from build123d import *

# Parameters (mm, degrees)
SKETCH1_W           = 25.4
SKETCH1_H           = 69.85
SKETCH1_R           = 3.175
BOSS_EXTRUDE1_DEPTH = 6.35
FILLET1_R           = 12.7
FILLET2_R           = 2.116666667
SKETCH5_R           = 9.525
SKETCH5_R_2         = 7.016807895
CUT_EXTRUDE2_DEPTH  = 3.571875
SKETCH5_2_R         = 7.016807895
CUT_EXTRUDE3_DEPTH  = 6.35


with BuildPart() as part:
    # Sketch1 → Boss-Extrude1 (new body)
    with BuildSketch(Plane(origin=(0, 0, 0), x_dir=(1, 0, 0), z_dir=(0, 1, 0))):
        Rectangle(SKETCH1_W, SKETCH1_H)
        with Locations(Location((0, -3.175, 0), (0, 0, 270))):
            Circle(SKETCH1_R, mode=Mode.SUBTRACT)
        with Locations(Location((0, -22.225, 0), (0, 0, 270))):
            Circle(SKETCH1_R, mode=Mode.SUBTRACT)
    extrude(amount=BOSS_EXTRUDE1_DEPTH)

    # Fillet1
    fillet1_edges = [part.edges().sort_by_distance(p)[0] for p in [
        (-12.7, 3.175, -34.925),
        (12.7, 3.175, -34.925),
        (-12.7, 3.175, 34.925),
        (12.7, 3.175, 34.925),
    ]]
    fillet(fillet1_edges, radius=FILLET1_R - 0.0001)  # a hair under: the kernel refuses the full size

    # Fillet2
    fillet2_edges = [part.edges().sort_by_distance(p)[0] for p in [
        (-12.7, 0, 0),
        (-12.7, 6.35, 0),
        (12.7, 0, 0),
        (8.98028541, 0, 31.20528541),
        (-8.98028541, 0, 31.20528541),
        (8.98028541, 0, -31.20528541),
        (-8.98028541, 0, -31.20528541),
        (12.7, 6.35, 0),
        (8.98028541, 6.35, 31.20528541),
        (-8.98028541, 6.35, 31.20528541),
        (8.98028541, 6.35, -31.20528541),
        (-8.98028541, 6.35, -31.20528541),
    ]]
    fillet(fillet2_edges, radius=FILLET2_R)

    # Sketch5 → Cut-Extrude2 (cut)
    with BuildSketch(Plane(origin=(0, 6.35, 0), x_dir=(1, 0, 0), z_dir=(0, 1, 0))):
        with Locations(Location((0, 22.225, 0), (0, 0, 270))):
            Circle(SKETCH5_R)
        with Locations(Location((0, 22.225, 0), (0, 0, 270))):
            Circle(SKETCH5_R_2, mode=Mode.SUBTRACT)
    extrude(amount=-CUT_EXTRUDE2_DEPTH, mode=Mode.SUBTRACT)

    # Sketch5<2> → Cut-Extrude3 (cut)
    with BuildSketch(Plane(origin=(0, 6.35, 0), x_dir=(1, 0, 0), z_dir=(0, 1, 0))):
        with Locations(Location((0, 22.225, 0), (0, 0, 270))):
            Circle(SKETCH5_2_R)
    extrude(amount=-CUT_EXTRUDE3_DEPTH, mode=Mode.SUBTRACT)


solid = part.part
Verification items for the finished model (mm, model axes). A direction names the side the tool comes from. Give positions to 0.01 mm unless a question says otherwise; leave off trailing zeros. Order: outer loops, then holes, each group sorted by start corner. A loop starts at its lowest first (then second) coordinate and runs counter-clockwise, first axis right, second up. Notation, with made-up numbers: M -12.5,-25 L -5.5,-25 A30 cw -5.5,3 Z; hole C 49.5,6 d6. An arc over 180 degrees is marked long. Answer as a JSON object with one key per item and string values. Group by question number.
1) Cross-section at A-A (y = 1). Give the number of separate pieces and of enclosed holes in the cut face, then the cut area to 3 significant figures.
2) Mould release check, pull along X, two halves, no side actions. Record for faces 1 (the face through (12.7, 3, 0)), 2 (the face through (-12.1, 0.64, -0.31)), 3 (the face through (0.309, 1.409, -29.235)): released by +X, released by -X, zero draft, split by the parting line, or undercut.
3) Scan lines: line 1 along Z through (x, y) = (-0.5, 4.75); line 2 along Z through (x, y) = (-6.25, 2); line 3 along Y through (x, z) = (10.5, -24.5). Record each from-to range of solid material in increasing order. Write a range as [from, to].
4) Cross-section at B-B (z = -19). Enter the section's corners in (x, y), then the cut area to 3 significant figures.
5) Cross-section at C-C (z = -11.5). Enter the section's corners in (x, y), then the cut area to 3 significant figures.
6) Access from +Z, -Z, +X, -X, +Y, -Y to the whole of each face (thin tool, end or side, straight path). Record for faces 4 (the face through (-6, 2.778, -27)), 5 (the face through (-12.1, 5.71, -0.31)).
7) Depth check by flat-ended pin: pin 1 Ø1 at (y, z) = (2.5, 27) entering from -X; pin 2 Ø2 at (x, y) = (8.5, 1) entering from +Z; pin 3 Ø3 at (x, y) = (4.5, 2.5) entering from +Z. Enter the tip coordinate at first touch or a pass-through.
Result sheet:
{
 "1": {"separate pieces": "1", "enclosed holes": "3", "area": "1,360 mm2"},
 "2": {"face 1": "released by +X", "face 2": "released by -X", "face 3": "undercut"},
 "3": {"line 1": "z = [-34.85, -31.74], [-12.71, 0.04], [6.31, 19.09], [25.36, 34.85]", "line 2": "z = [-33.28, -25.41], [-19.04, 33.28]", "line 3": "y = [0.01, 6.34]"},
 "4": {"outline": "M -12.7,2.12 A2.12 ccw -10.58,0 L -6.23,0 L -6.23,2.78 L -8.96,2.78 L -8.96,6.35 L -10.58,6.35 A2.12 ccw -12.7,4.23 Z; M 6.23,0 L 10.58,0 A2.12 ccw 12.7,2.12 L 12.7,4.23 A2.12 ccw 10.58,6.35 L 8.96,6.35 L 8.96,2.78 L 6.23,2.78 Z", "area": "58.8 mm2"},
 "5": {"outline": "M -12.7,2.12 A2.12 ccw -10.58,0 L 10.58,0 A2.12 ccw 12.7,2.12 L 12.7,4.23 A2.12 ccw 10.58,6.35 L -10.58,6.35 A2.12 ccw -12.7,4.23 Z", "area": "157 mm2"},
 "6": {"face 4": "+Y", "face 5": "+Z, -Z, -X, +Y"},
 "7": {"pin 1": "stops at x = -11.96", "pin 2": "stops at z = 32.26", "pin 3": "stops at z = 34.57"}
}
